Study the drawing (mm; zero at the part's minimum x, y, z) and answer. A direction names the side the tool comes from. Round coordinates to 2 decimals unless told otherwise and drop trailing zeros. Write each loop counter-clockwise with the first axis right and the second up, starting at its lowest first coordinate (ties: lowest second). Pieces come first, ordered by that corner, then holes.
(1) For the marked faces 1 and 2, determine the directions among +Z, -Z, +X, -X, +Y, -Y from which every point of the face is accessible in a straight line to the end or side of a thin tool.
(2) A cutting plane is placed at A-A, the plane y = 25. Give the vertices of the cut face in (x, z) (1 decimal), and give its area (3 significant figures).
(3) A cutting plane is placed at C-C, the plane z = 8. Give the number of separate pieces and of enclosed holes in the cut face, and give its area (3 significant figures).
(4) Find the intervals of material crossed by probe 1 along X at (y, z) = (25, 7.9) (1 decimal); probe 2 along Y at (x, z) = (82.5, 2); probe 3 along Z at (x, y) = (10, 25.5), in increasing order.
(5) Each of these flat-tipped pins is pushed along its axis until it touches: pin 1 Ø10.5 at (x, y) = (60.5, 3.5) entering from -Z; pin 2 Ø8 at (x, y) = (65.5, 21.5) entering from -Z; pin 3 Ø3.5 at (x, y) = (25.87, 25) entering from -Z; pin 4 Ø2 at (x, y) = (43.5, 25.5) entering from +Z. Where does it stop, or does it pass through?
(6) A cutting plane is placed at D-D, the plane x = 17.5. Give the vertices of the cut face in (y, z), and give its area (3 significant figures).
(7) A cutting plane is placed at B-B, the plane x = 27. Give the vertices of the cut face in (y, z).
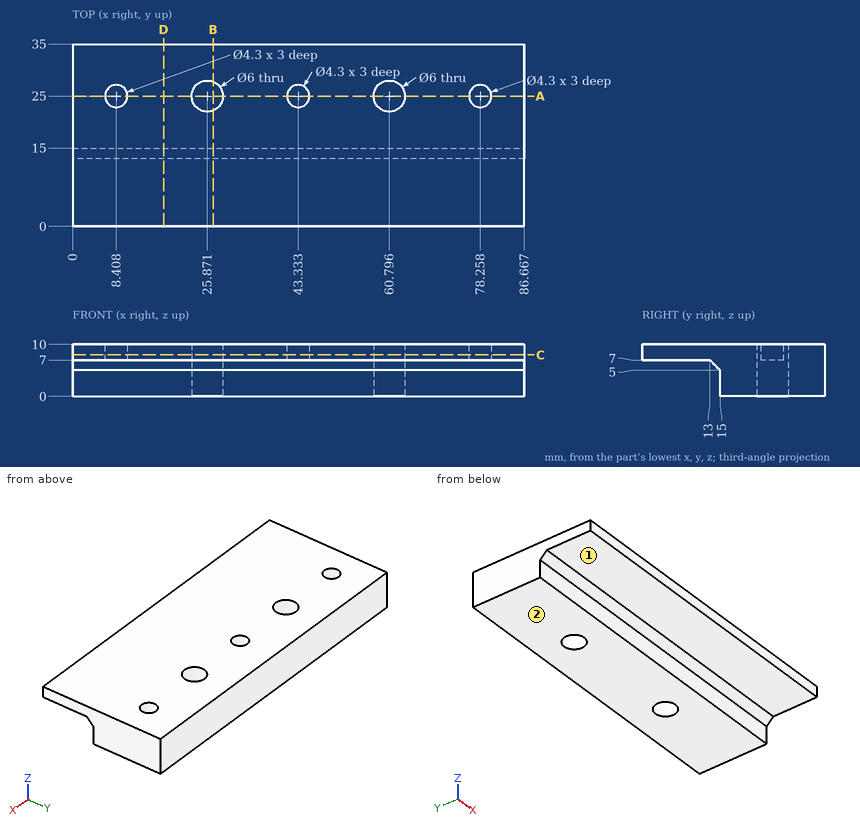
Solutions:
1. face 1: -Z, +X, -X, -Y
1. face 2: -Z, +X, -X, +Y, -Y
2. outline: (0, 0) - (22.9, 0) - (22.9, 10) - (10.6, 10) - (10.6, 7) - (6.3, 7) - (6.3, 10) - (0, 10) - close; (28.9, 0) - (57.8, 0) - (57.8, 10) - (45.5, 10) - (45.5, 7) - (41.2, 7) - (41.2, 10) - (28.9, 10) - close; (63.8, 0) - (86.7, 0) - (86.7, 10) - (80.4, 10) - (80.4, 7) - (76.1, 7) - (76.1, 10) - (63.8, 10) - close
2. area: 708 mm2
3. separate pieces: 1
3. enclosed holes: 5
3. area: 2,930 mm2
4. probe 1: x = 0 to 6.3, 10.6 to 22.9, 28.9 to 41.2, 45.5 to 57.8, 63.8 to 76.1, 80.4 to 86.7
4. probe 2: y = 15 to 35
4. probe 3: z = 0 to 7
5. pin 1: stops at z = 7
5. pin 2: stops at z = 0
5. pin 3: passes through
5. pin 4: stops at z = 7
6. outline: (0, 7) - (13, 7) - (15, 5) - (15, 0) - (35, 0) - (35, 10) - (0, 10) - close
6. area: 247 mm2
7. outline: (0, 7) - (13, 7) - (15, 5) - (15, 0) - (22.22, 0) - (22.22, 10) - (0, 10) - close; (27.78, 0) - (35, 0) - (35, 10) - (27.78, 10) - close
